The listing builds one solid part. Answer for the finished solid, in the listing's coordinates (mm). A direction names the side the tool comes from. Give positions to 0.01 mm unless a question says otherwise; leave off trailing zeros. Loops run counter-clockwise (first coordinate to the right, second up) from the corner with the lowest first, then second, coordinate; pieces in that order, holes last. Notation, with made-up numbers: M 19,86.25 L 74,86.25 A34 ccw 74,122.25 Z; hole C 66.5,31.25 d1. An arc over 180 degrees is marked long. Return JSON: item names as keys, results as strings.
from build123d import *

# Parameters (mm, degrees)
SKETCH_1_R      = 1.45
EXTRUDE_1_DEPTH = 2
FILLET_1_R      = 5
FILLET_2_R      = 3


with BuildPart() as part:
    # 草图1 → 凸台-拉伸1 (new body)
    with BuildSketch(Plane(origin=(0, 0, 0), x_dir=(1, 0, 0), z_dir=(0, 1, 0))):
        Polygon((207.315214967, -87.759054481), (201.010915634, -101.369925501), (230, -114.797123874), (245, -114.797123874), (245, -111.623574981), (245, -71.122908945), (230, -71.122908945), align=None)
        with Locations(Location((217.77393632, -100.868789323, 0), (0, 0, 270))):
            Circle(SKETCH_1_R, mode=Mode.SUBTRACT)
        with Locations(Location((208.700022307, -96.665923102, 0), (0, 0, 270))):
            Circle(SKETCH_1_R, mode=Mode.SUBTRACT)
        with Locations(Location((237.5, -86.122908945, 0), (0, 0, 270))):
            Circle(SKETCH_1_R, mode=Mode.SUBTRACT)
        with Locations(Location((237.5, -76.122908945, 0), (0, 0, 270))):
            Circle(SKETCH_1_R, mode=Mode.SUBTRACT)
        Polygon((230, -77.323350324), (230, -98.266220035), (212.497179662, -90.159243016), align=None, mode=Mode.SUBTRACT)
    extrude(amount=EXTRUDE_1_DEPTH)

    # 圆角1
    fillet_1_edges = [part.edges().sort_by_distance(p)[0] for p in [
        (230, 1, 71.122908945),
        (245, 1, 71.122908945),
        (245, 1, 114.797123874),
        (230, 1, 114.797123874),
        (201.010915634, 1, 101.369925501),
        (207.315214967, 1, 87.759054481),
    ]]
    fillet(fillet_1_edges, radius=FILLET_1_R)

    # 圆角2
    fillet_2_edges = [part.edges().sort_by_distance(p)[0] for p in [
        (230, 1, 77.323350324),
        (212.497179662, 1, 90.159243016),
        (230, 1, 98.266220035),
    ]]
    fillet(fillet_2_edges, radius=FILLET_2_R)


solid = part.part
(1) Determine the mould class of faces 1 (the flat face through (236, 1, 71.123)), 2 (the flat face through (235, 1, 114.797)), 3 (the cylindrical face through (207.285, 0.986, 96.352)) for opening direction Z: released by +Z, released by -Z, zero draft, split by the parting line, or undercut.
Values follow:
{"face 1": "released by -Z", "face 2": "released by +Z", "face 3": "undercut"}
(2) Straight lines are drawn through the part: line 1 along Z through (x, y) = (237.5, 0.6); line 2 along Z through (x, y) = (238, 0.1); line 3 along Z through (x, y) = (220.5, 0.75). For each, find the intervals that lie inside material, in ascending order.
Values follow:
{"line 1": "71.12 to 74.67, 77.57 to 84.67, 87.57 to 114.8", "line 2": "71.12 to 74.76, 77.48 to 84.76, 87.48 to 114.8", "line 3": "78.09 to 84.29, 93.87 to 110.4"}
(3) Given pin 1 (1 mm diameter, centred on x = 240, z = 107.5, fed in from -Y); pin 2 (1 mm diameter, centred on y = 1.5, z = 103, fed in from -X); pin 3 (0.6 mm diameter, centred on y = 1, z = 87.5, fed in from -X), each flat-ended and moving along its own axis, determine where each tip first touches the part or whether it passes through.
Values follow:
{"pin 1": "y = 0", "pin 2": "x = 204.14", "pin 3": "x = 207.49"}
(4) The part is cut by section A-A (x = 237.5). Determine the outline of the cut face in (y, z), and give its area (3 significant figures).
Values follow:
{"outline": "M 0,71.12 L 2,71.12 L 2,74.67 L 0,74.67 Z; M 0,77.57 L 2,77.57 L 2,84.67 L 0,84.67 Z; M 0,87.57 L 2,87.57 L 2,114.8 L 0,114.8 Z", "area": "75.7 mm²"}
(5) The part is cut by section B-B (y = 0.4). Determine the outline of the cut face in (x, z).
Values follow:
{"outline": "M 203.11,96.83 L 206.77,88.93 A5 ccw 208.35,87 L 228.68,72.09 A5 ccw 231.64,71.12 L 240,71.12 A5 ccw 245,76.12 L 245,109.8 A5 ccw 240,114.8 L 231.1,114.8 A5 ccw 229,114.33 L 205.55,103.47 A5 ccw Z; hole C 208.7,96.67 d2.9; hole C 217.77,100.87 d2.9; hole M 216.6,87.15 L 225.23,80.82 A3 ccw 230,83.24 L 230,93.57 A3 ccw 225.74,96.29 L 217.11,92.3 A3 ccw Z; hole C 237.5,76.12 d2.9; hole C 237.5,86.12 d2.9"}
(6) A tool of negligible diameter and unlimited length cuts with its end or side. For faces 4 (the flat face through (245, 1, 93)), 5 (the flat face through (221.48, 0.99, 94.32)), from which of +Z, -Z, +X, -X, +Y, -Y can it reach the whole face along a straight path? Write none if from no direction.
Values follow:
{"face 4": "+Z, -Z, +X, +Y, -Y", "face 5": "+Y, -Y"}
